Check sheet for the modelled part. Datum: model origin and axes. Units: mm. Face numbers are marked on the shaded views. A direction names the side the tool comes from. Round coordinates to 2 decimals unless told otherwise and drop trailing zeros. Order: outer loops, then holes, each group sorted by start corner. A loop starts at its lowest first (then second) coordinate and runs counter-clockwise, first axis right, second up. Notation, with made-up numbers: M 22.25,21 L 52.25,21 A22 cw 52.25,29 Z; hole C 4,17.25 d1. An arc over 180 degrees is marked long. One line per item, written item: value. Start each with the question number.
(1) Cross-section at B-B, the plane z = 7.5. Enter the section's corners in (x, y).
(2) Release check for a two-part mould opening along Y. For the marked faces 1, 2, 3 and 4 record: released by +Y, released by -Y, zero draft, split by the parting line, or undercut.
(3) Thickness scan on L1, parallel to Y at x = -7.5, z = 7.25; L2, parallel to Y at x = 10, z = 2.45; L3, parallel to Y at x = -6.5, z = 4.25. Record the ranges inside material, lowest first.
(4) Cross-section at D-D, the plane y = -1.05. Enter the section's corners in (x, z), and give its area (3 significant figures).
(5) Access from +Z, -Z, +X, -X, +Y, -Y to the whole of each face (thin tool, end or side, straight path). Record for the marked faces 5, 6, 7 and 8.
(6) Cross-section at A-A, the plane y = 15. Enter the section's corners in (x, z), and give its area (3 significant figures).
(7) Cross-section at C-C, the plane x = 10. Enter the section's corners in (y, z), and give its area (3 significant figures).
(8) Depth check by flat-ended pin: pin 1 Ø1.3 at (x, z) = (-8.5, 7) entering from +Y; pin 2 Ø1 at (x, y) = (-7.5, 13.45) entering from +Z; pin 3 Ø4 at (x, z) = (-9, 5.5) entering from -Y; pin 4 Ø7 at (x, y) = (-7.5, 4.95) entering from -Z. Enter the tip coordinate at first touch or a pass-through.
from build123d import *

# Parameters (mm, degrees)
ESQUISSE1_R             = 2.05
BOSS_EXTRU_1_DEPTH      = 4
BOSS_EXTRU_2_DEPTH      = 4.5
ESQUISSE3_R             = 0.85
ENL_V_MAT_EXTRU_1_DEPTH = 8
CONG_1_R                = 2.5


with BuildPart() as part:
    # Esquisse1 → Boss.-Extru.1 (new body)
    with BuildSketch(Plane.XY):
        Polygon((0, 20), (20, 20), (20, -20), (0, -20), (-1, -16), (-16, -16), (-16, 16), (-1, 16), align=None)
        with Locations((10, 15)):
            Circle(ESQUISSE1_R, mode=Mode.SUBTRACT)
        with Locations((10, -15)):
            Circle(ESQUISSE1_R, mode=Mode.SUBTRACT)
        with BuildLine():
            ThreePointArc((-10.40473751, -0.3), (-7.5, 10.95), (-4.59526249, -0.3))
            ThreePointArc((-4.59526249, -0.3), (-7.5, -4.05), (-10.40473751, -0.3))
        make_face(mode=Mode.SUBTRACT)
    extrude(amount=BOSS_EXTRU_1_DEPTH)

    # Esquisse2 → Boss.-Extru.2 (add)
    with BuildSketch(Plane.XY.offset(4)):
        with BuildLine():
            Line((-0.1, -13.5), (-0.1, 13.5))
            ThreePointArc((-0.1, 13.5), (-0.832233047, 15.267766953), (-2.6, 16))
            Line((-2.6, 16), (-16, 16))
            Line((-16, 16), (-16, -16))
            Line((-16, -16), (-2.6, -16))
            ThreePointArc((-2.6, -16), (-0.832233047, -15.267766953), (-0.1, -13.5))
        make_face()
        Polygon((-1.5, 4.950000005), (-1.5, -12.05), (-13.5, -12.05), (-13.5, 4.95), (-13.5, 10.95), (-7.499999947, 10.95), (-1.5, 10.95), align=None, mode=Mode.SUBTRACT)
    extrude(amount=BOSS_EXTRU_2_DEPTH)

    # Esquisse3 → Enlèv. mat.-Extru.1 (cut)
    with BuildSketch(Plane.XY.offset(8.5)):
        with Locations((-7.5, 13.45)):
            Circle(ESQUISSE3_R)
        with Locations((-7.5, -14.55)):
            Circle(ESQUISSE3_R)
    extrude(amount=-ENL_V_MAT_EXTRU_1_DEPTH, mode=Mode.SUBTRACT)

    # Congé1
    cong_1_edges = [part.edges().sort_by_distance(p)[0] for p in [
        (-16, -16, 4.25),
        (-16, 16, 4.25),
        (0, 20, 2),
        (20, 20, 2),
        (20, -20, 2),
        (0, -20, 2),
    ]]
    fillet(cong_1_edges, radius=CONG_1_R)


solid = part.part
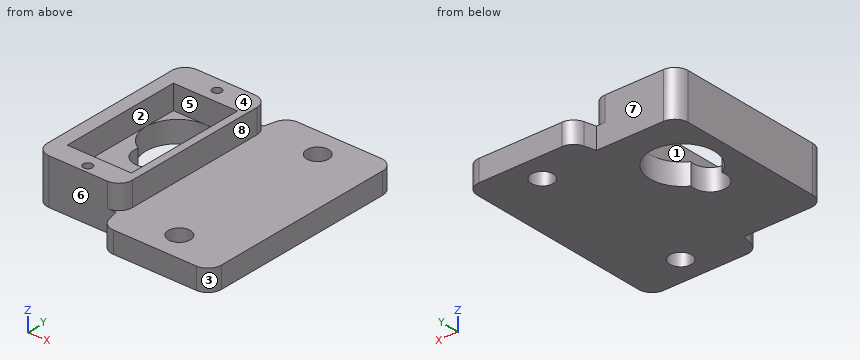
Values found:
1. outline: M -16,-13.5 A2.5 ccw -13.5,-16 L -2.6,-16 A2.5 ccw -0.1,-13.5 L -0.1,13.5 A2.5 ccw -2.6,16 L -13.5,16 A2.5 ccw -16,13.5 Z; hole M -13.5,-12.05 L -1.5,-12.05 L -1.5,10.95 L -13.5,10.95 Z; hole C -7.5,-14.55 d1.7; hole C -7.5,13.45 d1.7
2. face 1: undercut
2. face 2: undercut
2. face 3: released by -Y
2. face 4: zero draft
3. L1: -16 to -15.4, -13.7 to -12.05, 10.95 to 12.6, 14.3 to 16
3. L2: -20 to -17.05, -12.95 to 12.95, 17.05 to 20
3. L3: -16 to -12.05, 10.95 to 16
4. outline: M -16,0 L -10.5,0 L -10.5,4 L -13.5,4 L -13.5,8.5 L -16,8.5 Z; M -4.5,0 L 20,0 L 20,4 L -0.1,4 L -0.1,8.5 L -1.5,8.5 L -1.5,4 L -4.5,4 Z
4. area: 138 mm^2
5. face 5: +Z
5. face 6: +Z, -Z, -X, -Y
5. face 7: +Z, -Z, -X, +Y
5. face 8: +Z, +X, +Y, -Y
6. outline: M -15.5,0 L 7.95,0 L 7.95,4 L -0.6,4 L -0.6,8.5 L -15.5,8.5 Z; M 12.05,0 L 20,0 L 20,4 L 12.05,4 Z
6. area: 193 mm^2
7. outline: M -20,0 L -17.05,0 L -17.05,4 L -20,4 Z; M -12.95,0 L 12.95,0 L 12.95,4 L -12.95,4 Z; M 17.05,0 L 20,0 L 20,4 L 17.05,4 Z
7. area: 127 mm^2
8. pin 1: y = 16
8. pin 2: z = 0.5
8. pin 3: y = -16
8. pin 4: through
